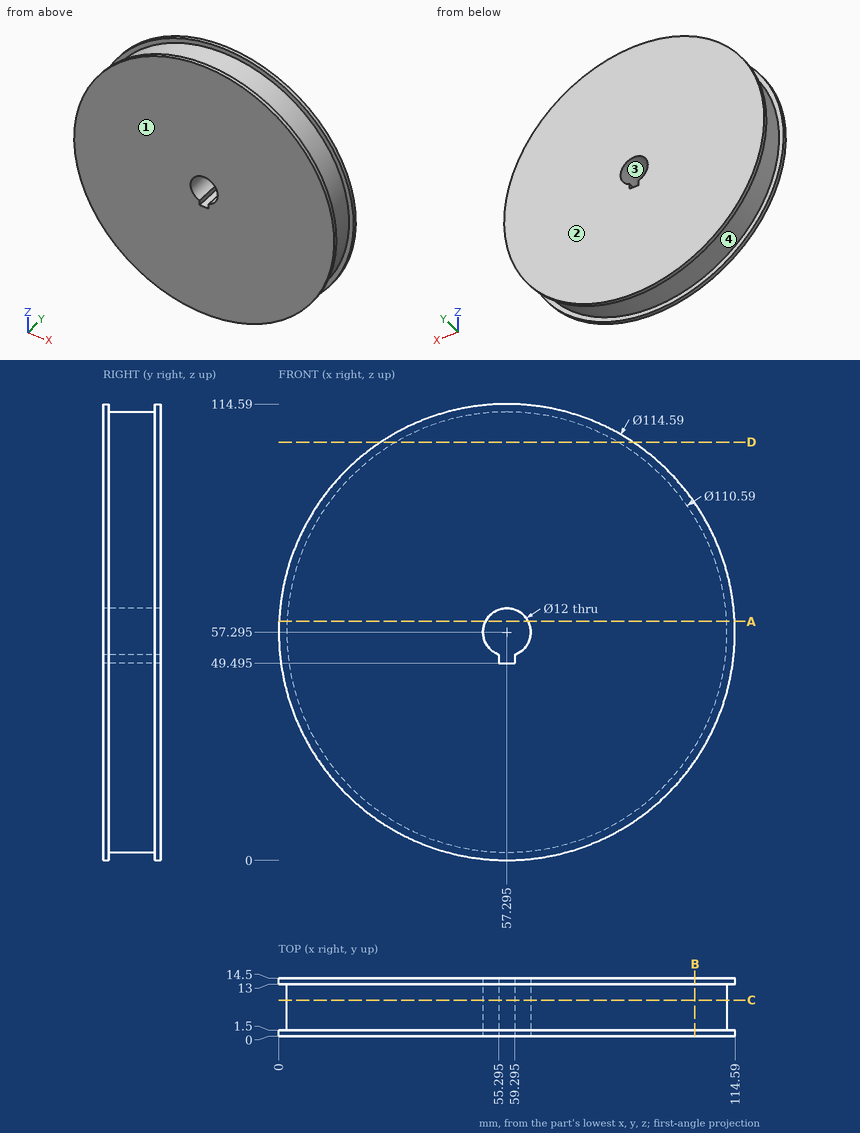
Drawing for the job (mm, zero at the part's lowest x, y, z). Give positions to 0.01 mm unless a question says otherwise; leave off trailing zeros. Order: outer loops, then holes, each group sorted by start corner. A loop starts at its lowest first (then second) coordinate and runs counter-clockwise, first axis right, second up. Notation, with made-up numbers: M 39.25,41.25 L 62.25,41.25 A31 cw 62.25,79.25 Z; hole C 21.25,87.25 d1. An arc over 180 degrees is marked long. Use a Markdown table: item, result. Add a question column.
(1) Saw through at A-A, the plane z = 60. Give the cut face in (x, y).
(2) Drop flat-ended pins along their axis: P1, Ø8, axis at y = 9.5, z = 99, coming from the -X side; P2, Ø6, axis at y = 12.5, z = 43.5, coming from the +X side; P3, Ø3, axis at y = 11, z = 59, coming from the -X side. Give the stop position or say it passes through.
(3) Saw through at B-B, the plane x = 104.5. Give the cut face in (y, z), and give its area (3 significant figures).
(4) Saw through at D-D, the plane z = 105. Give the cut face in (x, y), and give its area (3 significant figures).
(5) Mould opens along Y. For the marked faces 1, 2, 3 and 4 say: +Y half, -Y half, draft (parallel to the pull), parting line (faces both ways), or undercut.
(6) Probe line 1 along Z through (x, y) = (62, 9.25); line 2 along X through (y, z) = (4, 19); line 3 along X through (y, z) = (3, 53.5). List the from-to ranges inside material, lowest first. Write a range as [from, to].
(7) Saw through at C-C, the plane y = 9. Give the cut face in (x, z) (3 decimals), and give its area (3 significant figures).
Answer key:
| question | item | result |
|---|---|---|
| 1 | outline | M 0.06,0 L 51.94,0 L 51.94,14.5 L 0.06,14.5 L 0.06,13 L 2.07,13 L 2.07,1.5 L 0.06,1.5 Z; M 62.65,0 L 114.53,0 L 114.53,1.5 L 112.52,1.5 L 112.52,13 L 114.53,13 L 114.53,14.5 L 62.65,14.5 Z |
| 2 | P1 | x = 16.05 |
| 2 | P2 | x = 113.56 |
| 2 | P3 | x = 2 |
| 3 | outline | M 0,24.82 L 1.5,24.82 L 1.5,28.5 L 13,28.5 L 13,24.82 L 14.5,24.82 L 14.5,89.77 L 13,89.77 L 13,86.09 L 1.5,86.09 L 1.5,89.77 L 0,89.77 Z |
| 3 | area | 857 mm^2 |
| 4 | outline | M 25.56,0 L 89.03,0 L 89.03,1.5 L 85.26,1.5 L 85.26,13 L 89.03,13 L 89.03,14.5 L 25.56,14.5 L 25.56,13 L 29.33,13 L 29.33,1.5 L 25.56,1.5 Z |
| 4 | area | 833 mm^2 |
| 5 | face 1 | -Y half |
| 5 | face 2 | +Y half |
| 5 | face 3 | draft |
| 5 | face 4 | undercut |
| 6 | line 1 | [2.2, 53.57], [61.02, 112.39] |
| 6 | line 2 | [17.41, 97.18] |
| 6 | line 3 | [2.13, 52.65], [61.94, 112.46] |
| 7 | outline | C 57.295,57.295 d110.59; hole M 55.295,49.495 L 59.295,49.495 L 59.295,51.638 A6 ccw long 55.295,51.638 Z |
| 7 | area | 9,480 mm^2 |
